Could you check a few things on this model? Use its own coordinates, in mm. Coordinates: 2 decimals unless noted, no trailing zeros. Order: outer loops, then holes, each group sorted by start corner. A loop starts at its lowest first (then second) coordinate and runs counter-clockwise, first axis right, second up. Notation, with made-up numbers: M 28,75.25 L 41,75.25 A26 ccw 41,90.25 Z; hole C -31.5,61.25 d4. An arc over 180 degrees is marked long. Write item = value, one per line. Start each with the question number.
from build123d import *

# Parameters (mm, degrees)
BOSS_EXTRUDE1_DEPTH = 406.4
SKETCH2_W           = 239.802769694
SKETCH2_H           = 6.35
CUT_EXTRUDE1_DEPTH  = 6.35
SKETCH3_W           = 223.774
SKETCH3_H           = 6.35
CUT_EXTRUDE2_DEPTH  = 2.3622
CAVITY1_START       = 6.35
CAVITY1_OUTLINE_W   = 86.976200951
CAVITY1_OUTLINE_H   = 12.7
CAVITY1_DEPTH       = 6.35


# Read off the part's stored shape, not the designer's step: Cavity1
with BuildPart() as part:
    # Sketch1 → Boss-Extrude1 (new body)
    with BuildSketch(Plane.XY):
        Polygon((0, 0), (5.260512242, 12.7), (223.774, 12.7), (223.774, 0), align=None)
    extrude(amount=BOSS_EXTRUDE1_DEPTH)

    # Sketch2 → Cut-Extrude1 (cut)
    with BuildSketch(Plane.XZ.offset(-12.7)):
        with Locations((97.522615153, 3.175)):
            Rectangle(SKETCH2_W, SKETCH2_H)
    extrude(amount=CUT_EXTRUDE1_DEPTH, mode=Mode.SUBTRACT)

    # Sketch3 → Cut-Extrude2 (cut)
    with BuildSketch(Plane.XZ.offset(-12.7)):
        with Locations((111.887, 403.225)):
            Rectangle(SKETCH3_W, SKETCH3_H)
    extrude(amount=CUT_EXTRUDE2_DEPTH, mode=Mode.SUBTRACT)

    # Cavity1 outline → Cavity1 (cut)
    with BuildSketch(Plane(origin=(0, 0, 0), x_dir=(1, 0, 0), z_dir=(0, 1, 0)).offset(CAVITY1_START)):
        with Locations((77.210447741, -203.2)):
            Rectangle(CAVITY1_OUTLINE_W, CAVITY1_OUTLINE_H)
    extrude(amount=CAVITY1_DEPTH, mode=Mode.SUBTRACT)


solid = part.part
(1) Imagine slicing it at A-A on x = 55.5. List the corners of the cut face in (y, z) for me, plus the area to 3 significant figures.
(2) Thinking about a two-plate mould opening in Z: for faces 1 (the flat face through (2.593, 6.261, 200.355)), 2 (the flat face through (113, 4, 0)), 3 (the flat face through (77, 6.35, 203)), which applies, released by +Z, released by -Z, zero draft, split by the parting line, or undercut?
(3) Will these pins go through, and if not, where does the flat tip stop? P1, Ø7, axis at y = 9, z = 2, coming from the -X side; P2, Ø7, axis at x = 126, y = 10, coming from the -Z side; P3, Ø3, axis at x = 101.5, z = 404, coming from the +Y side.
(4) Please list where these lines run through material, in increasing order: probe 1 along Z at (x, y) = (97.5, 9); probe 2 along Z at (x, y) = (93.5, 12.25); probe 3 along Z at (x, y) = (131.5, 10.75). Write a range as from..to.
Response:
q1.outline = M 0,0 L 6.35,0 L 6.35,6.35 L 12.7,6.35 L 12.7,196.85 L 6.35,196.85 L 6.35,209.55 L 12.7,209.55 L 12.7,400.05 L 10.34,400.05 L 10.34,406.4 L 0,406.4 Z
q1.area = 5,030 mm2
q2.face_1 = zero draft
q2.face_2 = released by -Z
q2.face_3 = undercut
q3.P1 = 2.28
q3.P2 = 6.35
q3.P3 = 10.34
q4.probe_1 = 6.35..196.85, 209.55..406.4
q4.probe_2 = 6.35..196.85, 209.55..400.05
q4.probe_3 = 6.35..400.05
